Print and shaded views of the part. All mm, measured from the part's lowest x, y and z. Round coordinates to 2 decimals unless told otherwise and drop trailing zeros. Order: outer loops, then holes, each group sorted by start corner. A loop starts at its lowest first (then second) coordinate and runs counter-clockwise, first axis right, second up. Notation, with made-up numbers: (47, 83.25) -> (59, 83.25) arc R7 cw to (59, 92.25) -> close; hole circle Ø4 at (12.5, -32.75). An arc over 180 degrees is marked (long way). Answer as CSV lines item,"result".
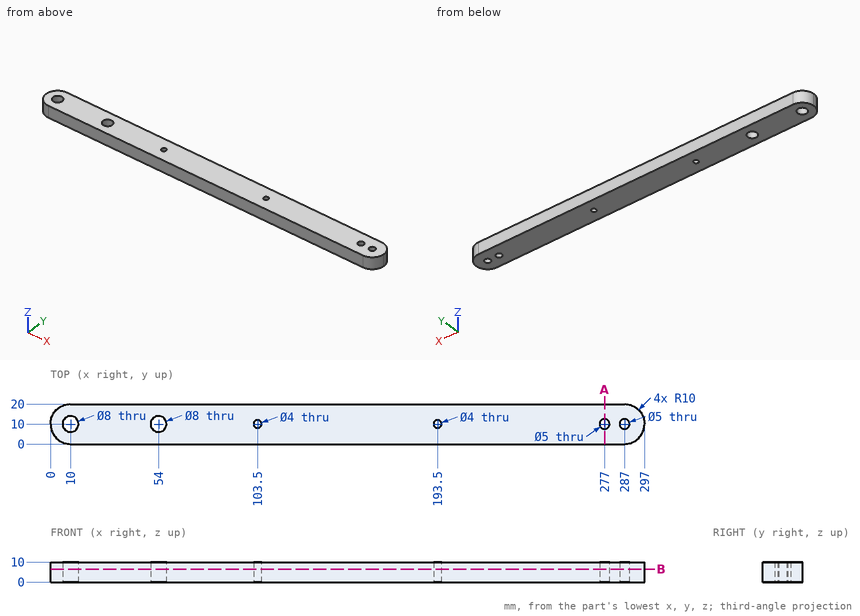
Q1. Wall check: L1, parallel to Y at x = 287, z = 2; L2, parallel to X at y = 12.25, z = 1; L3, parallel to X at y = 15.25, z = 6.75. Give the ranges that are in metal, low to high. Write a range as [from, to].
Checks:
L1,"[0, 7.5], [12.5, 20]"
L2,"[0.26, 6.69], [13.31, 50.69], [57.31, 275.91], [278.09, 285.91], [288.09, 296.74]"
L3,"[1.49, 295.51]"
Q2. Flat gauge pin, fed straight in: pin 1 (1.5 mm diameter, centred on y = 11, z = 5.5, fed in from +X). Where does the tip first touch, or does it go through?
Checks:
pin 1,"x = 297"
Q3. Saw through at A-A (x = 277). Write the cut outline in (y, z), plus the area to 3 significant figures.
Checks:
outline,"(0, 0) -> (7.5, 0) -> (7.5, 10) -> (0, 10) -> close; (12.5, 0) -> (20, 0) -> (20, 10) -> (12.5, 10) -> close"
area,"150 mm²"
Q4. Saw through at B-B (z = 6.5). State how many separate pieces and enclosed holes the cut face has, plus the area to 3 significant figures.
Checks:
separate pieces,"1"
enclosed holes,"6"
area,"5,690 mm²"
